from build123d import *

# Parameters (mm, degrees)
SKETCH1_W                        = 203.2
SKETCH1_H                        = 304.8
BOSS_EXTRUDE1_DEPTH              = 9.525
CUT_EXTRUDE1_REACH               = 185.41
SKETCH2_R                        = 20.574
CUT_EXTRUDE2_REACH               = 185.41
SKETCH3_W                        = 203.2
SKETCH3_H                        = 63.5
F_1_4_20_TAPPED_HOLE1_AT_2_COUNT = 2
F_1_4_20_TAPPED_HOLE1_AT_2_PITCH = 25.4
CUT_EXTRUDE3_REACH               = 137.338
SKETCH6_W                        = 50.8
SKETCH6_H                        = 177.8


with BuildPart() as part:
    # Sketch1 → Boss-Extrude1 (new body)
    with BuildSketch(Plane.XY):
        Rectangle(SKETCH1_W, SKETCH1_H)
    extrude(amount=BOSS_EXTRUDE1_DEPTH)

    # Sketch2 → Cut-Extrude1 (cut, up to next)
    with BuildSketch(Plane.XY.offset(9.525), mode=Mode.PRIVATE) as cut_extrude1_sk1:
        Circle(SKETCH2_R)
    cut_extrude1_tool1 = extrude(cut_extrude1_sk1.sketch, amount=-CUT_EXTRUDE1_REACH, mode=Mode.PRIVATE) & part.part
    add(cut_extrude1_tool1.solids().sort_by_distance((0, 0, 9.525))[0], mode=Mode.SUBTRACT)

    # Sketch3 → Cut-Extrude2 (cut, up to next)
    with BuildSketch(Plane.XY.offset(9.525), mode=Mode.PRIVATE) as cut_extrude2_sk1:
        with Locations((0, -120.65)):
            Rectangle(SKETCH3_W, SKETCH3_H)
    cut_extrude2_tool1 = extrude(cut_extrude2_sk1.sketch, amount=-CUT_EXTRUDE2_REACH, mode=Mode.PRIVATE) & part.part
    # Sketch3 → Cut-Extrude2 (cut, up to next)
    with BuildSketch(Plane.XY.offset(9.525), mode=Mode.PRIVATE) as cut_extrude2_sk2:
        with Locations((0, 120.65)):
            Rectangle(SKETCH3_W, SKETCH3_H)
    cut_extrude2_tool2 = extrude(cut_extrude2_sk2.sketch, amount=-CUT_EXTRUDE2_REACH, mode=Mode.PRIVATE) & part.part
    add(cut_extrude2_tool1.solids().sort_by_distance((0, -120.65, 9.525))[0], mode=Mode.SUBTRACT)
    add(cut_extrude2_tool2.solids().sort_by_distance((0, 120.65, 9.525))[0], mode=Mode.SUBTRACT)

    # Sketch5 → 1/4-20 Tapped Hole1 (revolve, cut)
    with BuildSketch(Plane(origin=(-12.7, 88.9, 4.7625), x_dir=(0, 0, 1), z_dir=(1, 0, 0))):
        Polygon((0, 0), (0, 20.583816902), (2.5527, 19.05), (2.5527, 0), align=None)
    f_1_4_20_tapped_hole1 = revolve(axis=Axis((-12.7, 95.25, 4.7625), (0, -1, 0)), mode=Mode.SUBTRACT)

    # 1/4-20 Tapped Hole1 at 2: 1/4-20 Tapped Hole1 ×2
    with Locations(*[(i * F_1_4_20_TAPPED_HOLE1_AT_2_PITCH, 0, 0) for i in range(1, F_1_4_20_TAPPED_HOLE1_AT_2_COUNT)]):
        add(f_1_4_20_tapped_hole1, mode=Mode.SUBTRACT)

    # Mirror1: 1/4-20 Tapped Hole1 across plane
    add(f_1_4_20_tapped_hole1.mirror(Plane.ZX), mode=Mode.SUBTRACT)

    # Mirror1 copy 1 sketch → Mirror1 copy 1 (revolve, cut)
    with BuildSketch(Plane(origin=(12.7, -88.9, 4.7625), x_dir=(0, 0, 1), z_dir=(1, 0, 0))):
        Polygon((0, 0), (0, -20.583816902), (2.5527, -19.05), (2.5527, 0), align=None)
    revolve(axis=Axis((12.7, -95.25, 4.7625), (0, -1, 0)), mode=Mode.SUBTRACT)

    # Sketch6 → Cut-Extrude3 (cut, up to next)
    with BuildSketch(Plane.XY.offset(9.525), mode=Mode.PRIVATE) as cut_extrude3_sk1:
        with Locations((-76.2, 0)):
            Rectangle(SKETCH6_W, SKETCH6_H)
    cut_extrude3_tool1 = extrude(cut_extrude3_sk1.sketch, amount=-CUT_EXTRUDE3_REACH, mode=Mode.PRIVATE) & part.part
    # Sketch6 → Cut-Extrude3 (cut, up to next)
    with BuildSketch(Plane.XY.offset(9.525), mode=Mode.PRIVATE) as cut_extrude3_sk2:
        with Locations((76.2, 0)):
            Rectangle(SKETCH6_W, SKETCH6_H)
    cut_extrude3_tool2 = extrude(cut_extrude3_sk2.sketch, amount=-CUT_EXTRUDE3_REACH, mode=Mode.PRIVATE) & part.part
    add(cut_extrude3_tool1.solids().sort_by_distance((-76.2, 0, 9.525))[0], mode=Mode.SUBTRACT)
    add(cut_extrude3_tool2.solids().sort_by_distance((76.2, 0, 9.525))[0], mode=Mode.SUBTRACT)


solid = part.part
For this review, take the finished solid that the model builds, in its own axes (mm). A direction names the side the tool comes from. Round coordinates to 2 decimals unless told otherwise and drop trailing zeros. Write each loop counter-clockwise with the first axis right and the second up, starting at its lowest first coordinate (ties: lowest second). Pieces come first, ordered by that corner, then holes. Notation, with made-up numbers: (-18.75, 43.5) -> (32.25, 43.5) arc R7 cw to (32.25, 50.5) -> close; hole circle Ø10 at (-1, -14). An arc over 180 degrees is marked (long way). Use CSV: the item, a comma, the result in double quotes.
(1) For faces 5 (the face through (13.68, -79.51, 7.12)), 6 (the face through (-50.8, -1, 5)), 7 (the face through (-10.435, 79.508, 5.94)), list the 3-axis set-ups (+Z, -Z, +X, -X, +Y, -Y) from which the entire face can be reached by the end or side of a thin tool; tool diameter is ignored.
Computed values:
face 5,"-Y"
face 6,"+Z, -Z, -X, +Y, -Y"
face 7,"+Y"
(2) To check wall thickness, follow L1, parallel to Z at x = 12.7, y = -83.75 (3 decimals); L2, parallel to X at y = 10, z = 9; L3, parallel to Y at x = 17.5, z = 8.5. State the ranges of each line that lie inside material, in increasing order. Write a range as [from, to].
Computed values:
L1,"[0, 2.21], [7.315, 9.525]"
L2,"[-50.8, -17.98], [17.98, 50.8]"
L3,"[-88.9, -10.82], [10.82, 88.9]"
(3) Consider section B-B, the plane y = 0. Give the boundary of the cut face in (x, z) (3 decimals).
Computed values:
outline,"(-50.8, 0) -> (-20.574, 0) -> (-20.574, 9.525) -> (-50.8, 9.525) -> close; (20.574, 0) -> (50.8, 0) -> (50.8, 9.525) -> (20.574, 9.525) -> close"
(4) Draft analysis for pull direction Z (two halves, no side actions). For faces 1 (the face through (-1, 21, 9.525)), 2 (the face through (-13.14, -68.583, 4.705)), 3 (the face through (-1, 21, 0)), 4 (the face through (-2.68, 20.4, 4.83)), state which applies: +Z half, -Z half, draft (parallel to the pull), parting line (faces both ways), or undercut.
Computed values:
face 1,"+Z half"
face 2,"undercut"
face 3,"-Z half"
face 4,"draft"
(5) Consider section A-A, the plane x = 0. Give the boundary of the cut face in (y, z) (3 decimals), plus the area to 3 significant figures.
Computed values:
outline,"(-88.9, 0) -> (-20.574, 0) -> (-20.574, 9.525) -> (-88.9, 9.525) -> close; (20.574, 0) -> (88.9, 0) -> (88.9, 9.525) -> (20.574, 9.525) -> close"
area,"1,300 mm²"
(6) Clearance check with flat-ended pins moving along their axes: P1, Ø4, axis at x = -12.7, z = 4.76, coming from the +Y side; P2, Ø4.5, axis at x = 12.7, z = 4.76, coming from the -Y side. State where each tip first meets the part, or that it passes through.
Computed values:
P1,"y = 69.52"
P2,"y = -69.67"
